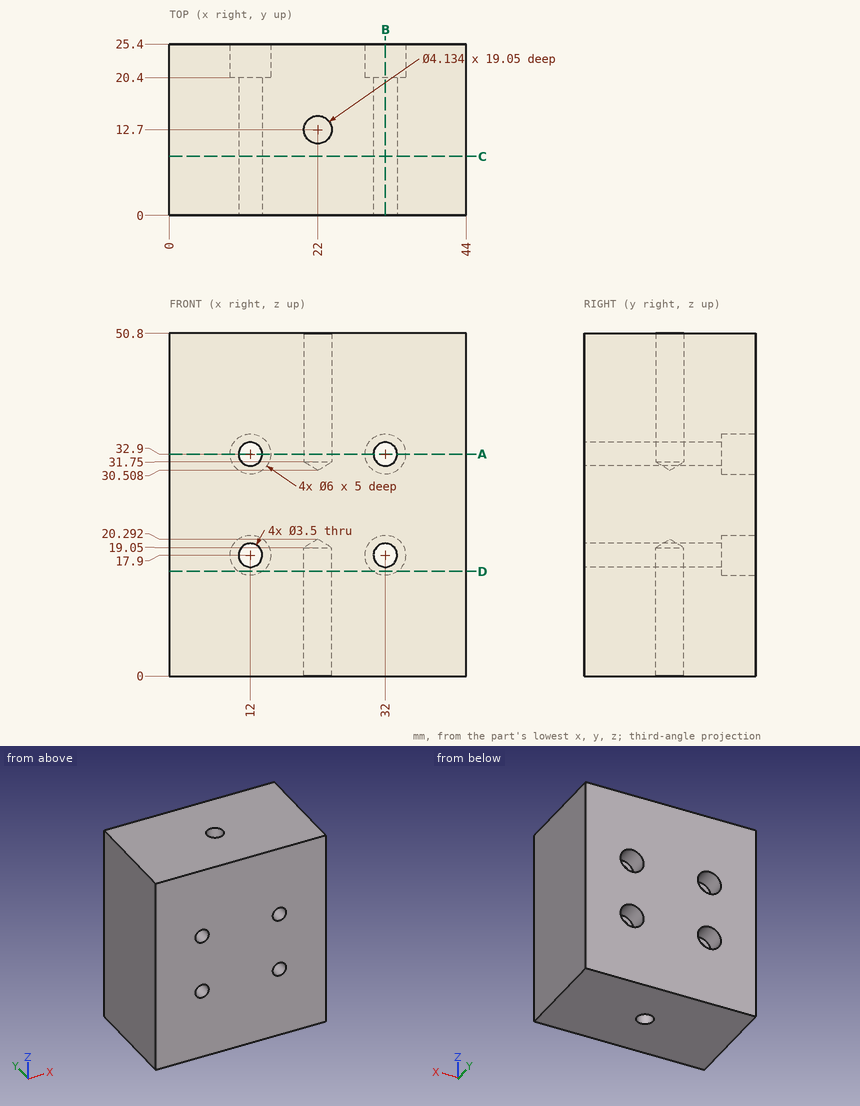
Design review of the part shown in the three views and the two pictorial views. Dimensions are in mm from the part's minimum x, y and z. Coordinates: 2 decimals unless noted, no trailing zeros. Order: outer loops, then holes, each group sorted by start corner. A loop starts at its lowest first (then second) coordinate and runs counter-clockwise, first axis right, second up. Notation, with made-up numbers: (26, -39) -> (33, -39) arc R37 cw to (33, 0) -> close; hole circle Ø5 at (80.5, 23.25). An arc over 180 degrees is marked (long way). Use one line per item in the form item = value. Start each with the question number.
(1) Add section B-B on x = 32. State the section outline as (y, z) points, plus the area to 3 significant figures.
(2) Add section D-D on z = 15.5. State the section outline as (x, y) points.
(3) Add section C-C on y = 8.75. State the section outline as (x, z) points, plus the area to 3 significant figures.
(4) Insertion check: pin 1 (3 mm diameter, centred on x = 31, z = 18.5, fed in from +Y); pin 2 (3 mm diameter, centred on x = 32, z = 17.9, fed in from -Y). Each pin has a flat end and moves straight along its axis. Give the tip position at first contact, or say it passes through.
(5) For probe 1 along X at (y, z) = (24, 32.9); probe 2 along Z at (x, y) = (12, 4.75); probe 3 along X at (y, z) = (6.75, 32.9), list the stretches that pass through material, from the lowest coordinate up.
(6) Add section A-A on z = 32.9. State the section outline as (x, y) points.
Answer block:
q1.outline = (0, 0) -> (25.4, 0) -> (25.4, 14.9) -> (20.4, 14.9) -> (20.4, 16.15) -> (0, 16.15) -> close; (0, 19.65) -> (20.4, 19.65) -> (20.4, 20.9) -> (25.4, 20.9) -> (25.4, 29.9) -> (20.4, 29.9) -> (20.4, 31.15) -> (0, 31.15) -> close; (0, 34.65) -> (20.4, 34.65) -> (20.4, 35.9) -> (25.4, 35.9) -> (25.4, 50.8) -> (0, 50.8) -> close
q1.area = 1,090 mm²
q2.outline = (0, 0) -> (44, 0) -> (44, 25.4) -> (33.8, 25.4) -> (33.8, 20.4) -> (30.2, 20.4) -> (30.2, 25.4) -> (13.8, 25.4) -> (13.8, 20.4) -> (10.2, 20.4) -> (10.2, 25.4) -> (0, 25.4) -> close; hole circle Ø4.13 at (22, 12.7)
q3.outline = (0, 0) -> (44, 0) -> (44, 50.8) -> (0, 50.8) -> close; hole circle Ø3.5 at (12, 17.9); hole circle Ø3.5 at (12, 32.9); hole circle Ø3.5 at (32, 17.9); hole circle Ø3.5 at (32, 32.9)
q3.area = 2,200 mm²
q4.pin_1 = 20.4
q4.pin_2 = through
q5.probe_1 = 0 to 9, 15 to 29, 35 to 44
q5.probe_2 = 0 to 16.15, 19.65 to 31.15, 34.65 to 50.8
q5.probe_3 = 0 to 10.25, 13.75 to 30.25, 33.75 to 44
q6.outline = (0, 0) -> (10.25, 0) -> (10.25, 20.4) -> (9, 20.4) -> (9, 25.4) -> (0, 25.4) -> close; (13.75, 0) -> (30.25, 0) -> (30.25, 20.4) -> (29, 20.4) -> (29, 25.4) -> (15, 25.4) -> (15, 20.4) -> (13.75, 20.4) -> close; (33.75, 0) -> (44, 0) -> (44, 25.4) -> (35, 25.4) -> (35, 20.4) -> (33.75, 20.4) -> close; hole circle Ø4.13 at (22, 12.7)
